Design review of the part shown in the three views and the two pictorial views. Dimensions are in mm from the part's minimum x, y and z. A direction names the side the tool comes from. Round coordinates to 2 decimals unless told otherwise and drop trailing zeros. Order: outer loops, then holes, each group sorted by start corner. A loop starts at its lowest first (then second) coordinate and runs counter-clockwise, first axis right, second up.
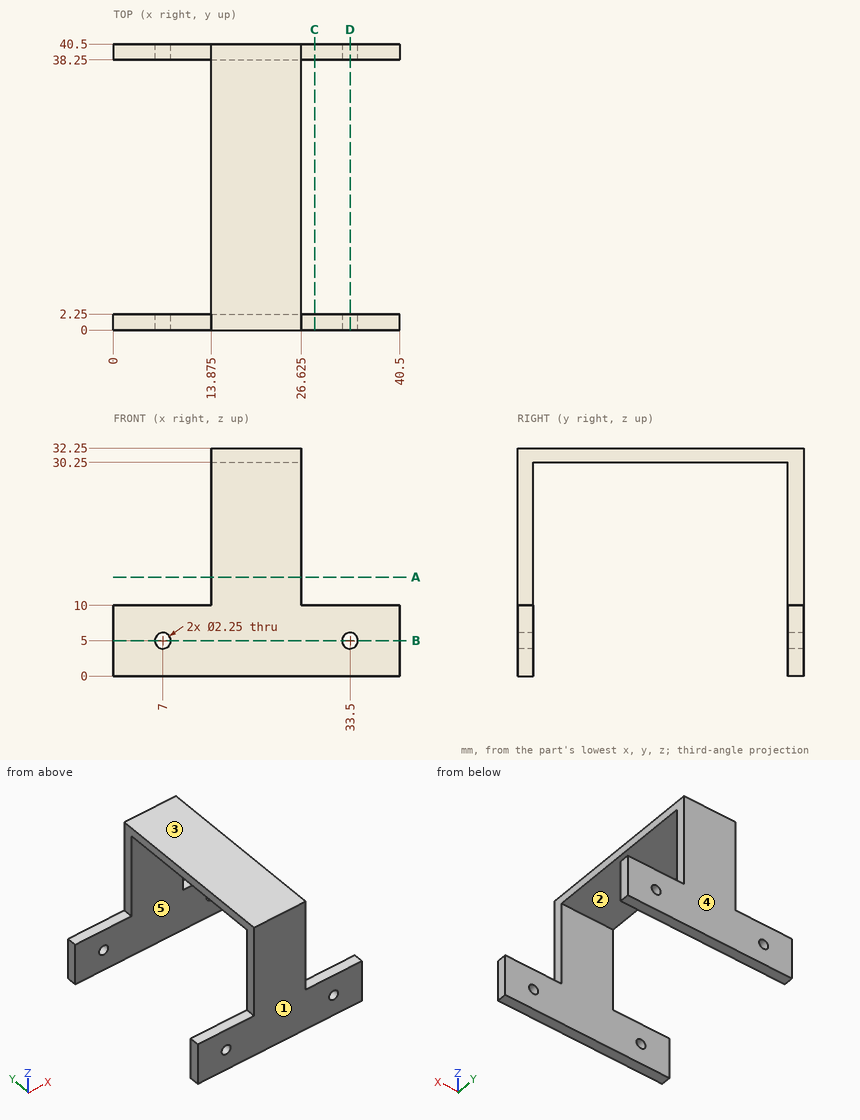
(1) For the marked faces 1 and 2, list the 3-axis set-ups (+Z, -Z, +X, -X, +Y, -Y) from which the entire face can be reached by the end or side of a thin tool; tool diameter is ignored.
Data:
face 1: +Z, -Z, +X, -X, -Y
face 2: -Z, +X, -X
(2) Consider section A-A (z = 14). Write out the cut boundary in (x, y) (3 decimals).
Data:
outline: (13.875, 0) - (26.625, 0) - (26.625, 2.25) - (13.875, 2.25) - close; (13.875, 38.25) - (26.625, 38.25) - (26.625, 40.5) - (13.875, 40.5) - close
(3) Draft analysis for pull direction Y (two halves, no side actions). For the marked faces 3, 4 and 5, state which applies: pulls with the +Y half, pulls with the -Y half, needs draft (parallel to the pull), parting line crosses it, or undercut.
Data:
face 3: needs draft
face 4: pulls with the +Y half
face 5: undercut
(4) Insertion check: pin 1 (4 mm diameter, centred on x = 21, y = 17, fed in from -Z); pin 2 (0.7 mm diameter, centred on x = 34.5, y = 1.5, fed in from +Z); pin 3 (2.5 mm diameter, centred on x = 7, z = 5, fed in from -Y); pin 4 (11 mm diameter, centred on y = 27.5, z = 26.5, fed in from +X) (3 decimals). Each pin has a flat end and moves straight along its axis. Give the tip position at first contact, or say it passes through.
Data:
pin 1: stops at z = 30.25
pin 2: stops at z = 10
pin 3: stops at y = 0
pin 4: stops at x = 26.625
(5) Consider section B-B (z = 5). Write out the cut boundary in (x, y) (3 decimals), and give its area (3 significant figures).
Data:
outline: (0, 0) - (5.875, 0) - (5.875, 2.25) - (0, 2.25) - close; (0, 38.25) - (5.875, 38.25) - (5.875, 40.5) - (0, 40.5) - close; (8.125, 0) - (32.375, 0) - (32.375, 2.25) - (8.125, 2.25) - close; (8.125, 38.25) - (32.375, 38.25) - (32.375, 40.5) - (8.125, 40.5) - close; (34.625, 0) - (40.5, 0) - (40.5, 2.25) - (34.625, 2.25) - close; (34.625, 38.25) - (40.5, 38.25) - (40.5, 40.5) - (34.625, 40.5) - close
area: 162 mm2
(6) Consider section D-D (x = 33.5). Write out the cut boundary in (y, z) (3 decimals), and give its area (3 significant figures).
Data:
outline: (0, 0) - (2.25, 0) - (2.25, 3.875) - (0, 3.875) - close; (0, 6.125) - (2.25, 6.125) - (2.25, 10) - (0, 10) - close; (38.25, 0) - (40.5, 0) - (40.5, 3.875) - (38.25, 3.875) - close; (38.25, 6.125) - (40.5, 6.125) - (40.5, 10) - (38.25, 10) - close
area: 34.9 mm2
(7) To check wall thickness, follow probe 1 along Z at (x, y) = (7, 39) (3 decimals); probe 2 along Y at (x, z) = (19, 21); probe 3 along Z at (x, y) = (24, 22.5). State the ranges of each line that lie inside material, in increasing order.
Data:
probe 1: z = 0 to 3.875, 6.125 to 10
probe 2: y = 0 to 2.25, 38.25 to 40.5
probe 3: z = 30.25 to 32.25
(8) Consider section C-C (x = 28.5). Write out the cut boundary in (y, z), and give its area (3 significant figures).
Data:
outline: (0, 0) - (2.25, 0) - (2.25, 10) - (0, 10) - close; (38.25, 0) - (40.5, 0) - (40.5, 10) - (38.25, 10) - close
area: 45.0 mm2
